Geometry check sheet. Reference: the model listing, model coordinates, mm. A direction names the side the tool comes from. Coordinates: 2 decimals unless noted, no trailing zeros. Write each loop counter-clockwise with the first axis right and the second up, starting at its lowest first coordinate (ties: lowest second). Pieces come first, ordered by that corner, then holes. Notation, with made-up numbers: (10.5, -21.75) -> (26.5, -21.75) arc R10 ccw to (26.5, -6.75) -> close; hole circle Ø7 at (-4, -27.5). An arc over 180 degrees is marked (long way). Answer in a Markdown table with one row per item. Add a question column.
Q1. Section check D-D, the plane y = 11. Record the boundary of the cut face in (x, z) (3 decimals), and give its area (4 significant figures).
Q2. Thickness scan on line 1 (Y direction, x = 4, z = 1.5); line 2 (Y direction, x = 11.5, z = 2.25); line 3 (Z direction, x = 9.5, y = 4.5). Record the ranges inside material, lowest first.
Q3. Tool access check on faces 4 (the face through (11.43, 31.009, 0.555)), 5 (the face through (9, 20, 3)). Record the directions out of +Z, -Z, +X, -X, +Y, -Y that give a thin tool (end or side, any length) a straight path to the whole face; none if there is none.
Q4. Section check A-A, the plane x = 4. Record the boundary of the cut face in (y, z), and give its area (3 significant figures).
Q5. Section check C-C, the plane z = 1.7. Record the boundary of the cut face in (x, y).
Q6. Section check B-B, the plane y = 20. Record the boundary of the cut face in (x, z).
Q7. Release check for a two-part mould opening along Y. For faces 1 (the face through (9, 20, 0)), 2 (the face through (11.43, 4.991, 0.555)), 3 (the face through (11, 40, 1)) record: pulls with the +Y half, pulls with the -Y half, needs draft (parallel to the pull), parting line crosses it, or undercut.
Q8. Gauge pin test, flat end, axial feed: P1, Ø1.6, axis at x = 4, y = 36, coming from the +Z side. Record the tip position at first contact, or that the pin passes through.
```python
from build123d import *

# Parameters (mm, degrees)
SKETCH1_W           = 23
SKETCH1_H           = 40
BOSS_EXTRUDE1_DEPTH = 3
SKETCH2_R           = 1.5
CUT_EXTRUDE1_DEPTH  = 4
CUT_EXTRUDE4_DEPTH  = 5
SKETCH4_R           = 1
CUT_EXTRUDE5_DEPTH  = 4


with BuildPart() as part:
    # Sketch1 → Boss-Extrude1 (new body)
    with BuildSketch(Plane.XY):
        with Locations((11.5, 20)):
            Rectangle(SKETCH1_W, SKETCH1_H)
    extrude(amount=BOSS_EXTRUDE1_DEPTH)

    # Sketch2 → Cut-Extrude1 (cut, through all)
    with BuildSketch(Plane.XY.offset(3)):
        with Locations((11.5, 20)):
            Circle(SKETCH2_R)
    extrude(amount=-CUT_EXTRUDE1_DEPTH, mode=Mode.SUBTRACT)

    # Sketch3 → Cut-Extrude4 (cut, symmetric)
    with BuildSketch(Plane(origin=(11.5, 0, 0), x_dir=(0, 0, -1), z_dir=(1, 0, 0))):
        with BuildLine():
            Line((0, 13.697030082), (0, 12.302969918))
            ThreePointArc((0, 12.302969918), (-0.029066134, 12.391711115), (-0.105, 12.446060799))
            ThreePointArc((-0.105, 12.446060799), (-0.175126488, 12.471018632), (-0.243202247, 12.501123596))
            ThreePointArc((-0.243202247, 12.501123596), (-0.555, 13), (-0.243202247, 13.498876404))
            ThreePointArc((-0.243202247, 13.498876404), (-0.175126488, 13.528981368), (-0.105, 13.553939201))
            ThreePointArc((-0.105, 13.553939201), (-0.029066134, 13.608288885), (0, 13.697030082))
        make_face()
        with BuildLine():
            Line((0, 11.697030082), (0, 10.302969918))
            ThreePointArc((0, 10.302969918), (-0.029066134, 10.391711115), (-0.105, 10.446060799))
            ThreePointArc((-0.105, 10.446060799), (-0.175126488, 10.471018632), (-0.243202247, 10.501123596))
            ThreePointArc((-0.243202247, 10.501123596), (-0.555, 11), (-0.243202247, 11.498876404))
            ThreePointArc((-0.243202247, 11.498876404), (-0.175126488, 11.528981368), (-0.105, 11.553939201))
            ThreePointArc((-0.105, 11.553939201), (-0.029066134, 11.608288885), (0, 11.697030082))
        make_face()
        with BuildLine():
            Line((0, 9.697030082), (0, 8.302969918))
            ThreePointArc((0, 8.302969918), (-0.029066134, 8.391711115), (-0.105, 8.446060799))
            ThreePointArc((-0.105, 8.446060799), (-0.175126488, 8.471018632), (-0.243202247, 8.501123596))
            ThreePointArc((-0.243202247, 8.501123596), (-0.555, 9), (-0.243202247, 9.498876404))
            ThreePointArc((-0.243202247, 9.498876404), (-0.175126488, 9.528981368), (-0.105, 9.553939201))
            ThreePointArc((-0.105, 9.553939201), (-0.029066134, 9.608288885), (0, 9.697030082))
        make_face()
        with BuildLine():
            Line((0, 7.697030082), (0, 6.302969918))
            ThreePointArc((0, 6.302969918), (-0.029066134, 6.391711115), (-0.105, 6.446060799))
            ThreePointArc((-0.105, 6.446060799), (-0.175126488, 6.471018632), (-0.243202247, 6.501123596))
            ThreePointArc((-0.243202247, 6.501123596), (-0.555, 7), (-0.243202247, 7.498876404))
            ThreePointArc((-0.243202247, 7.498876404), (-0.175126488, 7.528981368), (-0.105, 7.553939201))
            ThreePointArc((-0.105, 7.553939201), (-0.029066134, 7.608288885), (0, 7.697030082))
        make_face()
        with BuildLine():
            Line((0, 5.697030082), (0, 4.302969918))
            ThreePointArc((0, 4.302969918), (-0.029066134, 4.391711115), (-0.105, 4.446060799))
            ThreePointArc((-0.105, 4.446060799), (-0.175126488, 4.471018632), (-0.243202247, 4.501123596))
            ThreePointArc((-0.243202247, 4.501123596), (-0.555, 5), (-0.243202247, 5.498876404))
            ThreePointArc((-0.243202247, 5.498876404), (-0.175126488, 5.528981368), (-0.105, 5.553939201))
            ThreePointArc((-0.105, 5.553939201), (-0.029066134, 5.608288885), (0, 5.697030082))
        make_face()
        with BuildLine():
            Line((0, 3.697030082), (0, 2.302969918))
            ThreePointArc((0, 2.302969918), (-0.029066134, 2.391711115), (-0.105, 2.446060799))
            ThreePointArc((-0.105, 2.446060799), (-0.175126488, 2.471018632), (-0.243202247, 2.501123596))
            ThreePointArc((-0.243202247, 2.501123596), (-0.555, 3), (-0.243202247, 3.498876404))
            ThreePointArc((-0.243202247, 3.498876404), (-0.175126488, 3.528981368), (-0.105, 3.553939201))
            ThreePointArc((-0.105, 3.553939201), (-0.029066134, 3.608288885), (0, 3.697030082))
        make_face()
        with BuildLine():
            Line((0, 1.697030082), (0, 0.302969918))
            ThreePointArc((0, 0.302969918), (-0.029066134, 0.391711115), (-0.105, 0.446060799))
            ThreePointArc((-0.105, 0.446060799), (-0.175126488, 0.471018632), (-0.243202247, 0.501123596))
            ThreePointArc((-0.243202247, 0.501123596), (-0.555, 1), (-0.243202247, 1.498876404))
            ThreePointArc((-0.243202247, 1.498876404), (-0.175126488, 1.528981368), (-0.105, 1.553939201))
            ThreePointArc((-0.105, 1.553939201), (-0.029066134, 1.608288885), (0, 1.697030082))
        make_face()
    cut_extrude4 = extrude(amount=CUT_EXTRUDE4_DEPTH, both=True, mode=Mode.SUBTRACT)

    # Mirror1: Cut-Extrude4 across plane
    add(cut_extrude4.mirror(Plane(origin=(0, 20, 0), x_dir=(0, 0, 1), z_dir=(0, -1, 0))), mode=Mode.SUBTRACT)

    # Sketch4 → Cut-Extrude5 (cut, through all)
    with BuildSketch(Plane(origin=(0, 0, 0), x_dir=(-1, 0, 0), z_dir=(0, 0, -1))):
        with Locations((-19, 36)):
            Circle(SKETCH4_R)
        with Locations((-19, 4)):
            Circle(SKETCH4_R)
        with Locations((-4, 4)):
            Circle(SKETCH4_R)
        with Locations((-4, 36)):
            Circle(SKETCH4_R)
    extrude(amount=-CUT_EXTRUDE5_DEPTH, mode=Mode.SUBTRACT)


solid = part.part
```
Calculated:
| question | item | result |
|---|---|---|
| 1 | outline | (0, 0) -> (6.5, 0) -> (6.5, 0.555) -> (16.5, 0.555) -> (16.5, 0) -> (23, 0) -> (23, 3) -> (0, 3) -> close |
| 1 | area | 63.45 mm² |
| 2 | line 1 | y = 0 to 3, 5 to 35, 37 to 40 |
| 2 | line 2 | y = 0 to 18.5, 21.5 to 40 |
| 2 | line 3 | z = 0.24 to 3 |
| 3 | face 4 | -Z |
| 3 | face 5 | +Z, +X, -X, +Y, -Y |
| 4 | outline | (0, 0) -> (3, 0) -> (3, 3) -> (0, 3) -> close; (5, 0) -> (35, 0) -> (35, 3) -> (5, 3) -> close; (37, 0) -> (40, 0) -> (40, 3) -> (37, 3) -> close |
| 4 | area | 108 mm² |
| 5 | outline | (0, 0) -> (23, 0) -> (23, 40) -> (0, 40) -> close; hole circle Ø2 at (4, 4); hole circle Ø2 at (4, 36); hole circle Ø3 at (11.5, 20); hole circle Ø2 at (19, 4); hole circle Ø2 at (19, 36) |
| 6 | outline | (0, 0) -> (10, 0) -> (10, 3) -> (0, 3) -> close; (13, 0) -> (23, 0) -> (23, 3) -> (13, 3) -> close |
| 7 | face 1 | needs draft |
| 7 | face 2 | undercut |
| 7 | face 3 | pulls with the +Y half |
| 8 | P1 | passes through |
